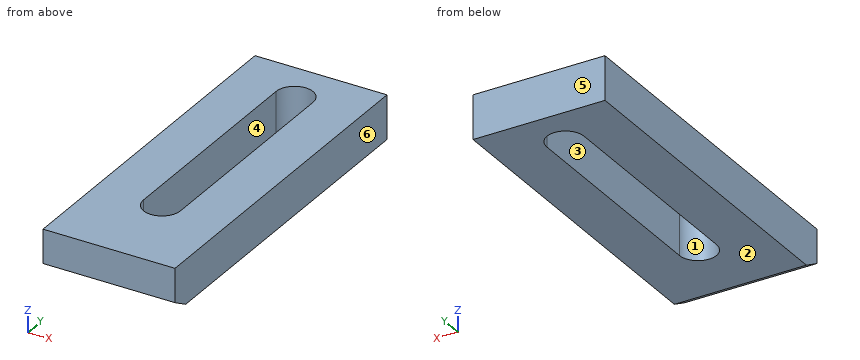
from build123d import *

# Parameters (mm, degrees)
SKETCH_1_W          = 75
SKETCH_1_H          = 200
EXTRUDE_1_DEPTH     = 25
CUT_EXTRUDE_1_DEPTH = 26
CHAMFER_1_SIZE      = 10
CHAMFER_1_SIZE2     = 5.773502692


with BuildPart() as part:
    # Эскиз1 → Бобышка-Вытянуть1 (new body)
    with BuildSketch(Plane.XY):
        with Locations((37.5, 100)):
            Rectangle(SKETCH_1_W, SKETCH_1_H)
    extrude(amount=EXTRUDE_1_DEPTH)

    # Эскиз2 → Вырез-Вытянуть1 (cut, through all)
    with BuildSketch(Plane.XY.offset(25)):
        with BuildLine():
            Line((27, 50), (27, 175))
            ThreePointArc((27, 175), (37.5, 185.5), (48, 175))
            Line((48, 175), (48, 50))
            ThreePointArc((48, 50), (37.5, 39.5), (27, 50))
        make_face()
    extrude(amount=-CUT_EXTRUDE_1_DEPTH, mode=Mode.SUBTRACT)

    # Фаска1
    chamfer_1_edges = [part.edges().sort_by_distance(p)[0] for p in [
        (37.5, 0, 0),
    ]]
    chamfer_1_side = [part.faces().sort_by_distance(p)[0] for p in [
        (37.5, 2.136000936, 0),
    ]]
    chamfer(chamfer_1_edges, length=CHAMFER_1_SIZE, length2=CHAMFER_1_SIZE2, reference=chamfer_1_side[0])


solid = part.part
Input: part model. Units: mm. Frame: model coordinates. Face numbers are marked on the shaded views. A direction names the side the tool comes from. Give positions to 0.01 mm unless a question says otherwise; leave off trailing zeros. Order: outer loops, then holes, each group sorted by start corner. A loop starts at its lowest first (then second) coordinate and runs counter-clockwise, first axis right, second up.
Q1. Ray query, probe 1 along X at (y, z) = (168, 19); probe 2 along Y at (x, z) = (36, 21.5); probe 3 along Y at (x, z) = (38.5, 22.75). Return the intervals inside material, ascending.
Checked values:
probe 1: x = 0 to 27, 48 to 75
probe 2: y = 0 to 39.61, 185.39 to 200
probe 3: y = 0 to 39.55, 185.45 to 200
Q2. Set-up query: the marked faces 1 and 2. Return all of +Z, -Z, +X, -X, +Y, -Y with unobstructed straight access to the full face (end or side cutting, diameter ignored); none if empty.
Checked values:
face 1: +Z, -Z
face 2: -Z, +X, -X, +Y, -Y
Q3. Section B-B on y = 170. Output: boundary loops of the cut face in (x, z), and give its area (3 significant figures).
Checked values:
outline: (0, 0) - (27, 0) - (27, 25) - (0, 25) - close; (48, 0) - (75, 0) - (75, 25) - (48, 25) - close
area: 1,350 mm2
Q4. Section A-A on x = 37.5. Output: boundary loops of the cut face in (y, z), and give its area (3 significant figures).
Checked values:
outline: (0, 5.77) - (10, 0) - (39.5, 0) - (39.5, 25) - (0, 25) - close; (185.5, 0) - (200, 0) - (200, 25) - (185.5, 25) - close
area: 1,320 mm2
Q5. Draft query along Y for the marked faces 3, 4, 5 and 6. Return one class per face: +Y half, -Y half, draft (parallel to the pull), parting line (faces both ways), or undercut.
Checked values:
face 3: undercut
face 4: undercut
face 5: +Y half
face 6: draft
